Autodesk Inventor part; units mm, degrees
ref_plane "YZ Plane" through (0, 0, 0) normal (1, 0, 0) x (0, 1, 0)
ref_plane "XZ Plane" through (0, 0, 0) normal (0, 1, 0) x (-1, 0, 0)
ref_plane "XY Plane" through (0, 0, 0) normal (0, 0, 1) x (1, 0, 0)
sketch "スケッチ1" plane through (0, 0, 0) normal (0, 0, 1) x (1, 0, 0)
  line L0 (-25, 25) -> (25, 25)
  line L1 (25, 25) -> (25, -25)
  line L2 (25, -25) -> (-25, -25)
  line L3 (-25, -25) -> (-25, 25)
  line L4 (-23, 23) -> (23, 23)
  line L5 (23, 23) -> (23, -23)
  line L6 (23, -23) -> (-23, -23)
  line L7 (-23, -23) -> (-23, 23)
  point P0 (0, 0)
  dimension "d0" = 50
  dimension "d1" = 50
  dimension "d2" = 46
  dimension "d3" = 46
  dimension "d4" = 25
  dimension "d5" = 23
  dimension "d142" = 23
  dimension "d143" = 25
extrude "押し出し1" add sketch "スケッチ1" along normal blind 150
sketch "スケッチ2" plane through (-25, 25, 0) normal (0, 1, 0) x (1, 0, 0)
  line L0 (0, 0) -> (50, 0)
  line L1 (0, 0) -> (0, -150)
  arc A0 (31, -32.5) -> (44, -32.5) centre (37.5, -32.5) ccw
  line L2 (31, -32.5) -> (31, 0)
  line L3 (44, -32.5) -> (44, 0)
  point P0 (25, 0)
  dimension "d10" = 13
  dimension "d11" = 32.5
  dimension "d12" = 37.5
extrude "押し出し2" cut sketch "スケッチ2" against normal blind 2
sketch "スケッチ3" plane through (-25, 25, 150) normal (0, 1, 0) x (1, 0, 0)
  arc A0 (31, 117.5) -> (44, 117.5) centre (37.5, 117.5) ccw
  circle A1 centre (29.5, 111) radius 1
  circle A2 centre (29.5, 147) radius 1
  circle A3 centre (45.5, 147) radius 1
  circle A4 centre (45.5, 111) radius 1
  point P0 (25, 150)
  dimension "d15" = 6.5
  dimension "d16" = 6.5
  dimension "d17" = 2
  dimension "d18" = 8
  dimension "d19" = 8
  dimension "d20" = 8
  dimension "d21" = 8
  dimension "d22" = 29.5
  dimension "d23" = 29.5
hole "穴1" at (4.5, 25, 3) at (20.5, 25, 3) at (20.5, 25, 39) at (4.5, 25, 39) direction (0, -1, 0) diameter 2 depth 2 tip angle 118 counterbore diameter 4 counterbore depth 0.5
sketch "スケッチ4" plane through (-25, -25, 0) normal (0, -1, 0) x (1, 0, 0)
  line L0 (50, 0) -> (0, 0)
  line L1 (50, 0) -> (50, 150)
  circle A0 centre (37.5, 9.5) radius 2
  point P0 (25, 0)
  dimension "d31" = 4
  dimension "d32" = 12.5
  dimension "d33" = 9.5
hole "穴2" at (12.5, -25, 9.5) direction (0, 1, 0) diameter 4 end through all
sketch "スケッチ7" plane through (-25, -25, 0) normal (0, -1, 0) x (1, 0, 0)
  line L0 (50, 0) -> (50, 150)
  circle A0 centre (37.5, 29) radius 4
  line L1 (50, 0) -> (0, 0)
  point P0 (25, 0)
  dimension "d79" = 8
  dimension "d80" = 12.5
  dimension "d88" = 29
hole "穴5" at (12.5, -25, 29) direction (0, 1, 0) diameter 8 end through all
sketch "スケッチ11" plane through (-25, -25, 0) normal (0, -1, 0) x (1, 0, 0)
  line L0 (50, 150) -> (0, 150)
  line L1 (50, 0) -> (50, 150)
  circle A0 centre (37.5, 140.5) radius 2
  point P0 (25, 0)
  dimension "d118" = 9.5
  dimension "d119" = 4
  dimension "d120" = 12.5
hole "穴7" at (12.5, -25, 140.5) direction (0, 1, 0) diameter 4 depth 2 tip angle 118
properties part number "07" material "アルミニウム 6061"
Verification items for the finished model (mm, model axes). A direction names the side the tool comes from. Give positions to 0.01 mm unless a question says otherwise; leave off trailing zeros. Order: outer loops, then holes, each group sorted by start corner. A loop starts at its lowest first (then second) coordinate and runs counter-clockwise, first axis right, second up. Notation, with made-up numbers: M 64,-22.5 L 122,-22.5 A24 ccw 122,-5.5 Z; hole C 49.5,-27 d2. An arc over 180 degrees is marked long. Return JSON: item names as keys, results as strings. Group by question number.
1) Section check A-A on x = 12.5. Record the cut outline in (y, z), and give its area (3 significant figures).
2) Access from +Z, -Z, +X, -X, +Y, -Y to the whole of each face (thin tool, end or side, straight path). Record for faces 4 (the face through (12.412, -23.986, 142.498)), 5 (the face through (14.9, -24, 32.2)), 6 (the face through (0, -23, 74)), 7 (the face through (4.412, 24.746, 37.002)).
3) Go/stop test with flat-tipped pins: pin 1 Ø1.8 at (x, z) = (4, 3.5) entering from +Y; pin 2 Ø2 at (x, z) = (11, 23) entering from +Y. Record where each tip stops, or that it passes through.
4) Section check B-B on y = 12. Record the cut outline in (x, z).
5) Mould release check, pull along Z, two halves, no side actions. Record for faces 1 (the face through (-2, -24, 150)), 2 (the face through (25, 0, 74)), 3 (the face through (18.517, 24.746, 38.74)): pulls with the +Z half, pulls with the -Z half, needs draft (parallel to the pull), parting line crosses it, or undercut.
6) Section check C-C on z = 29. Record the cut outline in (x, y), and give its area (3 significant figures).
7) Section check D-D on z = 109. Record the cut outline in (x, y).
8) Scan lines: line 1 (Z direction, x = 4.5, y = 24.9); line 2 (X direction, y = 23.3, z = 3); line 3 (Z direction, x = 4.5, y = 23.3). Record each from-to range of solid material in increasing order.
Answer block:
{
 "1": {"outline": "M -25,0 L -23,0 L -23,7.5 L -25,7.5 Z; M -25,11.5 L -23,11.5 L -23,25 L -25,25 Z; M -25,33 L -23,33 L -23,138.5 L -25,138.5 Z; M -25,142.5 L -23,142.5 L -23,150 L -25,150 Z; M 23,39 L 25,39 L 25,150 L 23,150 Z", "area": "490 mm^2"},
 "2": {"face 4": "-Y", "face 5": "+Y, -Y", "face 6": "+Z, -Z", "face 7": "+Y"},
 "3": {"pin 1": "stops at y = 24.5", "pin 2": "stops at y = -23"},
 "4": {"outline": "M -25,0 L -23,0 L -23,150 L -25,150 Z; M 23,0 L 25,0 L 25,150 L 23,150 Z"},
 "5": {"face 1": "pulls with the +Z half", "face 2": "needs draft", "face 3": "undercut"},
 "6": {"outline": "M -25,-25 L 8.5,-25 L 8.5,-23 L -23,-23 L -23,23 L 6,23 L 6,25 L -25,25 Z; M 16.5,-25 L 25,-25 L 25,25 L 19,25 L 19,23 L 23,23 L 23,-23 L 16.5,-23 Z", "area": "342 mm^2"},
 "7": {"outline": "M -25,-25 L 25,-25 L 25,25 L -25,25 Z; hole M -23,-23 L 23,-23 L 23,23 L -23,23 Z"},
 "8": {"line 1": "z = 0 to 1, 5 to 37, 41 to 150", "line 2": "x = -25 to 3.5, 5.5 to 6, 19 to 19.5, 21.5 to 25", "line 3": "z = 0 to 2, 4 to 38, 40 to 150"}
}
